```python
from build123d import *

# Parameters (mm, degrees)
SKETCH1_R           = 49.5046
BOSS_EXTRUDE1_DEPTH = 5.08
SKETCH2_R           = 47.625
BOSS_EXTRUDE2_DEPTH = 3.175
SKETCH3_R           = 6.731
SKETCH3_R_2         = 3.96875
SKETCH3_R_3         = 10
SKETCH3_R_4         = 2
SKETCH3_R_5         = 3.175
CUT_EXTRUDE1_DEPTH  = 9.255
SKETCH7_R           = 52.166274697
CUT_EXTRUDE4_DEPTH  = 5.08
SKETCH8_R           = 11.176
SKETCH8_R_2         = 6.35
CUT_EXTRUDE5_DEPTH  = 0.762


with BuildPart() as part:
    # Sketch1 → Boss-Extrude1 (new body)
    with BuildSketch(Plane.XY):
        Circle(SKETCH1_R)
    extrude(amount=BOSS_EXTRUDE1_DEPTH)

    # Sketch2 → Boss-Extrude2 (add)
    with BuildSketch(Plane.XY.offset(5.08)):
        Circle(SKETCH2_R)
    extrude(amount=BOSS_EXTRUDE2_DEPTH)

    # Sketch3 → Cut-Extrude1 (cut, through all)
    with BuildSketch(Plane.XY.offset(8.255)):
        with Locations((-12.7, -31.166793627)):
            Circle(SKETCH3_R)
        with Locations((12.7, -31.166793627)):
            Circle(SKETCH3_R)
        with Locations((-36.83, 0)):
            Circle(SKETCH3_R_2)
        with Locations((36.83, 0)):
            Circle(SKETCH3_R_2)
        with Locations((0, 6.35)):
            Circle(SKETCH3_R_3)
        with Locations((0, 28.326878759)):
            Circle(SKETCH3_R_4)
        with Locations((21.976878759, 6.35)):
            Circle(SKETCH3_R_4)
        with Locations((0, -15.626878759)):
            Circle(SKETCH3_R_4)
        with Locations((-21.976878759, 6.35)):
            Circle(SKETCH3_R_4)
        with Locations((-14.921345457, -10.968575281)):
            Circle(SKETCH3_R_5)
    extrude(amount=-CUT_EXTRUDE1_DEPTH, mode=Mode.SUBTRACT)

    # Sketch7 → Cut-Extrude4 (cut)
    with BuildSketch(Plane(origin=(0, 0, 0), x_dir=(-1, 0, 0), z_dir=(0, 0, -1))):
        Circle(SKETCH7_R)
    extrude(amount=-CUT_EXTRUDE4_DEPTH, mode=Mode.SUBTRACT)

    # Sketch8 → Cut-Extrude5 (cut)
    with BuildSketch(Plane(origin=(0, 0, 5.08), x_dir=(-1, 0, 0), z_dir=(0, 0, -1))):
        with Locations((-12.7, -31.166793627)):
            Circle(SKETCH8_R)
        with Locations((12.7, -31.166793627)):
            Circle(SKETCH8_R)
        with Locations((14.921345457, -10.968575281)):
            Circle(SKETCH8_R_2)
    extrude(amount=-CUT_EXTRUDE5_DEPTH, mode=Mode.SUBTRACT)


solid = part.part
```
For this review, take the finished solid that the model builds, in its own axes (mm). A direction names the side the tool comes from. Round coordinates to 2 decimals unless told otherwise and drop trailing zeros. Write each loop counter-clockwise with the first axis right and the second up, starting at its lowest first coordinate (ties: lowest second). Pieces come first, ordered by that corner, then holes. Notation, with made-up numbers: M -1,-12.5 L 26,-12.5 A33 ccw 26,22.5 Z; hole C 57,87 d7. An arc over 180 degrees is marked long. One line per item, written item: value. Start each with the question number.
(1) Machinability: for faces 1 (the cylindrical face through (0.923, -17.401, 6.69)), 2 (the cylindrical face through (-10.277, -42.077, 5.456)), which of the approach directions +Z, -Z, +X, -X, +Y, -Y give a long, thin tool a straight path to every point of the face, cutting with its end or side? Answer none if there is none.
(2) We need section A-A (x = 0). Give the boundary of the cut face in (y, z) (3 decimals).
(3) Wall thickness on line 1 (X direction, y = -35, z = 5.6); line 2 (Y direction, x = -14.5, z = 7.1); line 3 (Y direction, x = -14, z = 6.4): over which ranges is each line inside the solid? List them lowest first.
(4) Insertion check: pin 1 (6.5 mm diameter, centred on x = 36.83, y = 0, fed in from -Z). The pin has a flat end and moves straight along its axis. Give the tip position at first contact, or say it passes through.
(5) We need section D-D (z = 7.55). Count the separate pieces of the cut face and the enclosed holes in it, and give its area (3 significant figures).
(6) The part is to be moulded in two halves that separate along X. For faces 3 (the flat face through (-10, 1, 5.08)), 4 (the cylindrical face through (-2.17, -3.41, 6.69)), say which applies: released by +X, released by -X, zero draft, split by the parting line, or undercut.
(7) We need section B-B (x = 36.83). Give the boundary of the cut face in (y, z) (3 decimals).
(8) We need section C-C (y = 10). Give the boundary of the cut face in (x, z) (3 decimals), and give its area (3 significant figures).
Result:
1. face 1: +Z, -Z
1. face 2: -Z
2. outline: M -47.625,5.08 L -17.627,5.08 L -17.627,8.255 L -47.625,8.255 Z; M -13.627,5.08 L -3.65,5.08 L -3.65,8.255 L -13.627,8.255 Z; M 16.35,5.08 L 26.327,5.08 L 26.327,8.255 L 16.35,8.255 Z; M 30.327,5.08 L 47.625,5.08 L 47.625,8.255 L 30.327,8.255 Z
3. line 1: -32.3 to -23.2, -2.2 to 2.2, 23.2 to 32.3
3. line 2: -45.36 to -37.65, -24.68 to -14.12, -7.82 to 45.36
3. line 3: -45.52 to -37.77, -24.56 to -14.01, -7.93 to 45.52
4. pin 1: through
5. separate pieces: 1
5. enclosed holes: 10
5. area: 6,350 mm²
6. face 3: zero draft
6. face 4: undercut
7. outline: M -30.194,5.08 L -3.969,5.08 L -3.969,8.255 L -30.194,8.255 Z; M 3.969,5.08 L 30.194,5.08 L 30.194,8.255 L 3.969,8.255 Z
8. outline: M -46.563,5.08 L -9.31,5.08 L -9.31,8.255 L -46.563,8.255 Z; M 9.31,5.08 L 46.563,5.08 L 46.563,8.255 L 9.31,8.255 Z
8. area: 237 mm²
